```python
from build123d import *

# Parameters (mm, degrees)
F0_R     = 6.25
F1_DEPTH = 10


with BuildPart() as f1:
    # F0 (on Front) → F1 (new body)
    with BuildSketch(Plane.XZ):
        with BuildLine():
            Line((50, -58.640056), (17.56466, 0.924604))
            ThreePointArc((17.56466, 0.924604), (0, 11.359944), (-17.56466, 0.924604))
            Line((-17.56466, 0.924604), (-50, -58.640056))
            Line((-50, -58.640056), (-50, -108.640056))
            Line((-50, -108.640056), (0, -108.640056))
            Line((0, -108.640056), (50, -108.640056))
            Line((50, -108.640056), (50, -58.640056))
        make_face()
        with Locations((-25, -93.640056)):
            Circle(F0_R, mode=Mode.SUBTRACT)
        with Locations((-25, -68.640056)):
            Circle(F0_R, mode=Mode.SUBTRACT)
        with Locations((25, -93.640056)):
            Circle(F0_R, mode=Mode.SUBTRACT)
        with Locations((25, -68.640056)):
            Circle(F0_R, mode=Mode.SUBTRACT)
        with Locations((0, -8.640056)):
            Circle(F0_R, mode=Mode.SUBTRACT)
    extrude(amount=F1_DEPTH)


solid = f1.part
```
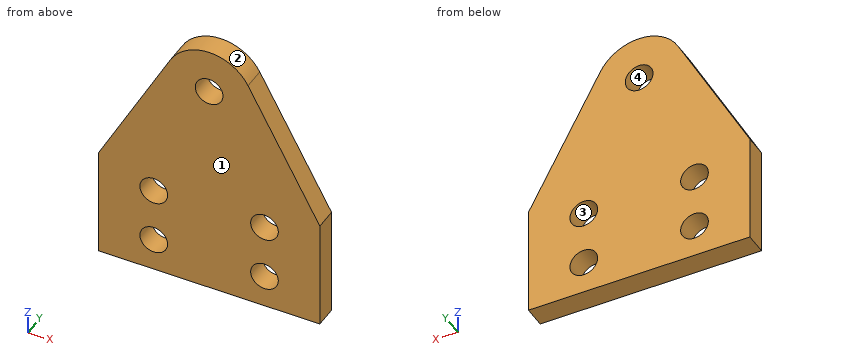
Check sheet for the modelled part. Datum: model origin and axes. Units: mm. Face numbers are marked on the shaded views. Round coordinates to 2 decimals unless told otherwise and drop trailing zeros. Write each loop counter-clockwise with the first axis right and the second up, starting at its lowest first coordinate (ties: lowest second). Pieces come first, ordered by that corner, then holes. Notation, with made-up numbers: M 72,73 L 122,73 A18 ccw 122,99 Z; hole C 41,28 d5. An arc over 180 degrees is marked long. Write item = value, one per line. Start each with the question number.
1. Section check C-C, the plane y = -3.5. Record the cut outline in (x, z).
2. Section check D-D, the plane x = 25. Record the cut outline in (y, z), then the cut area to 3 significant figures.
3. Scan lines: line 1 (X direction, y = -1.75, z = -63); line 2 (Z direction, x = 25, y = -7); line 3 (Z direction, x = -0.5, y = -0.5). Record each from-to range of solid material in increasing order. Write a range as [from, to].
4. Section check B-B, the plane z = -91. Record the cut outline in (x, y).
5. Gauge pin test, flat ends, axial feed: pin 1 (7.5 mm diameter, centred on x = 25, z = -93.64, fed in from -Y); pin 2 (6 mm diameter, centred on x = -11, y = -7, fed in from +Z). Record the tip position at first contact, or that the pin passes through.
6. Release check for a two-part mould opening along X. For the marked faces 1, 2, 3 and 4 record: pulls with the +X half, pulls with the -X half, needs draft (parallel to the pull), parting line crosses it, or undercut.
7. Section check A-A, the plane x = 0. Record the cut outline in (y, z), then the cut area to 4 significant figures.
Results found:
q1.outline = M -50,-108.64 L 50,-108.64 L 50,-58.64 L 17.56,0.92 A20 ccw -17.56,0.92 L -50,-58.64 Z; hole C -25,-93.64 d12.5; hole C -25,-68.64 d12.5; hole C 0,-8.64 d12.5; hole C 25,-93.64 d12.5; hole C 25,-68.64 d12.5
q2.outline = M -10,-108.64 L 0,-108.64 L 0,-99.89 L -10,-99.89 Z; M -10,-87.39 L 0,-87.39 L 0,-74.89 L -10,-74.89 Z; M -10,-62.39 L 0,-62.39 L 0,-12.73 L -10,-12.73 Z
q2.area = 709 mm^2
q3.line_1 = [-50, -27.69], [-22.31, 22.31], [27.69, 50]
q3.line_2 = [-108.64, -99.89], [-87.39, -74.89], [-62.39, -12.73]
q3.line_3 = [-108.64, -14.87], [-2.41, 11.35]
q4.outline = M -50,-10 L -30.67,-10 L -30.67,0 L -50,0 Z; M -19.33,-10 L 19.33,-10 L 19.33,0 L -19.33,0 Z; M 30.67,-10 L 50,-10 L 50,0 L 30.67,0 Z
q5.pin_1 = through
q5.pin_2 = 9.69
q6.face_1 = needs draft
q6.face_2 = parting line crosses it
q6.face_3 = undercut
q6.face_4 = undercut
q7.outline = M -10,-108.64 L 0,-108.64 L 0,-14.89 L -10,-14.89 Z; M -10,-2.39 L 0,-2.39 L 0,11.36 L -10,11.36 Z
q7.area = 1,075 mm^2
